Build history of the part. All positions in model axes, mm. Give positions to 0.01 mm unless a question says otherwise; leave off trailing zeros. Loops run counter-clockwise (first coordinate to the right, second up) from the corner with the lowest first, then second, coordinate; pieces in that order, holes last.
1) Wall check: line 1 (Y direction, x = 25.75, z = 3); line 2 (Y direction, x = 22.25, z = 6.25); line 3 (Z direction, x = 39, y = 70.75). Give the ranges that are in metal, low to high.
2) Band-saw the part on A-A on y = 71. List the corners of the cut face in (x, z), then the cut area to 3 significant figures.
3) Band-saw the part on B-B on z = 0. List the corners of the cut face in (x, y) (1 decimal).
4) Flat gauge pins, fed straight in: P1, Ø1, axis at x = 37, y = 72.5, coming from the +Z side; P2, Ø1, axis at x = 29, z = -4, coming from the +Y side; P3, Ø0.5, axis at y = 74.5, z = -11, coming from the -X side. Where does each tip first touch, or does it go through?
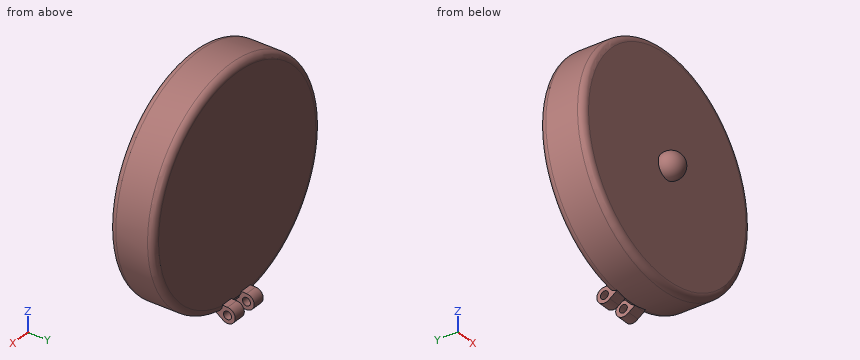
Autodesk Inventor part; units mm, degrees
ref_plane "Work Plane1" through (31.3182, 0, 0) normal (1, 0, 0) x (0, 1, 0)
ref_plane "XZ Plane" through (0, 0, 0) normal (0, 1, 0) x (-1, 0, 0)
ref_plane "XY Plane" through (0, 0, 0) normal (0, 0, 1) x (1, 0, 0)
sketch "Sketch1" plane through (0, 0, 0) normal (0, 0, 1) x (1, 0, 0)
  line L0 (8.9491, 93.5489) -> (53.3991, 93.5489) construction
  line L1 (53.3991, 93.5489) -> (53.3991, 10.9989) construction
  line L2 (53.3991, 10.9989) -> (8.9491, 10.9989) construction
  line L3 (8.9491, 10.9989) -> (8.9491, 93.5489) construction
  line L4 (42.5105, 69.6145) -> (42.5105, 74.0469)
  line L5 (31.1983, 74.0469) -> (31.1983, 69.6145)
  line L6 (31.1983, 74.0469) -> (42.5105, 74.0469)
  line L7 (42.5105, 69.6145) -> (31.1983, 69.6145)
  circle A0 centre (31.1983, 69.2335) radius 1.27
  line L8 (31.1983, 69.6145) -> (31.1983, 67.9635)
  point P0 (0, 0)
  point P1 (32.4098, 69.6145)
  dimension "d3" = 2.54
  dimension "d4" = 0.381
revolve "Revolution1" add sketch "Sketch1" angle 360 about axis through (31.1983, 74.0469, 0) along (0, -1, 0) contours L7 A0 L5 L6 L4 | A0 L8 L7 | L7 L5 A0
fillet "Fillet1" radius 0.635 2 edges at (19.8861, 74.0469, 0) (19.8861, 69.6145, 0)
ref_plane "Work Plane1" through (31.3182, 0, 0) normal (1, 0, 0) x (0, 1, 0)
sketch "Sketch3" plane through (31.3182, 0, 0) normal (1, 0, 0) x (0, 1, 0)
  line L0 (91.7474, 13.6776) -> (91.7474, -13.6861) construction
  line L1 (91.7474, -13.6861) -> (69.2257, -13.6861) construction
  line L2 (69.2257, -13.6861) -> (69.2257, 13.6776) construction
  line L3 (69.2257, 13.6776) -> (91.7474, 13.6776) construction
  circle A0 centre (74.5674, -11.1927) radius 0.765
  circle A1 centre (74.5674, -11.1927) radius 0.3969
  line L4 (74.033, -11.7401) -> (73.4119, -11.3003)
  line L5 (73.4119, -11.3122) -> (73.4119, 11.3122)
  line L6 (74.5674, -10.4276) -> (74.0469, -10.4034)
  line L7 (74.0469, 10.6772) -> (74.0469, -10.6772)
  line L8 (73.818, -11.0391) -> (73.4119, -11.3003)
  line L9 (74.0727, -10.4046) -> (72.7289, -10.3422)
  line L10 (72.7289, -10.3422) -> (73.4119, -11.3003)
  point P0 (0, 0)
  point P1 (74.0469, -10.632)
  dimension "d49" = 1.53
  dimension "d50" = 0.7937
extrude "Extrusion1" add sketch "Sketch3" along normal mid plane 3.81 contours A0
extrude "Extrusion2" cut sketch "Sketch3" along normal mid plane 1.3335 contours A0 | A1
extrude "Extrusion3" add sketch "Sketch3" along normal mid plane 3.81 contours A0 L7 L6 | L4 L8 A0 | A0 L8 L5 L9 L7 | L10 L9 L5
extrude "Extrusion4" cut sketch "Sketch3" along normal mid plane 1.3335 contours A0 L7 L6 | L4 L8 A0
properties part number "Neck_3DPrint"
Findings below:
1. line 1: y = 69.61 to 74.05
1. line 2: y = 69.66 to 74
1. line 3: z = -8.19 to 8.19
2. outline: circle Ø22.62 at (31.2, 0)
2. area: 402 mm2
3. outline: (19.9, 70.2) arc R0.6 ccw to (20.5, 69.6) - (30, 69.6) arc R1.3 ccw (long way) to (32.4, 69.6) - (41.9, 69.6) arc R0.6 ccw to (42.5, 70.2) - (42.5, 73.4) arc R0.6 ccw to (41.9, 74) - (20.5, 74) arc R0.6 ccw to (19.9, 73.4) - close
4. P1: stops at z = 9.99
4. P2: stops at y = 74.05
4. P3: stops at x = 29.41
